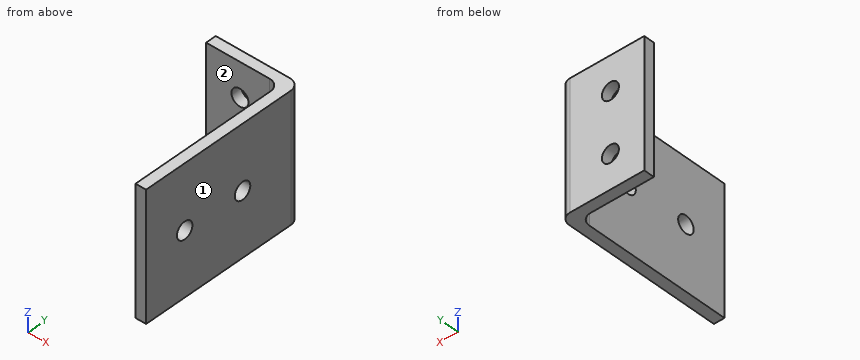
from build123d import *

# Parameters (mm, degrees)
F0_W     = 22.225
F0_H     = 38.1
F0_W_2   = 3.175
F1_DEPTH = 3.175
F2_D     = 5.1054
F3_DEPTH = 50.8
F4_R     = 3.175
F6_D     = 5.1054


with BuildPart() as f1:
    # F0 (on Front) → F1 (new body)
    with BuildSketch(Plane.XZ):
        with Locations((-0.7963004947, 15.9530722331)):
            Rectangle(F0_W, F0_H)
        with Locations((11.9036995053, 15.9530722331)):
            Rectangle(F0_W_2, F0_H)
    extrude(amount=F1_DEPTH)

    # F2 (through all)
    with Locations(Plane(origin=(0, 0, 0), x_dir=(1, 0, 0), z_dir=(0, 1, 0))):
        with Locations((-1.7488004947, -24.8430722331), (-1.7488004947, -7.0630722331)):
            Hole(F2_D / 2)

    # F0 (on Front) → F3 (join)
    with BuildSketch(Plane.XZ):
        with Locations((11.9036995053, 15.9530722331)):
            Rectangle(F0_W_2, F0_H)
    extrude(amount=F3_DEPTH)

    # F4
    f4_edges = [f1.edges().sort_by_distance(p)[0] for p in [
        (10.3162, -3.175, 15.953072),
        (13.4912, 0, 15.953072),
    ]]
    fillet(f4_edges, radius=F4_R)

    # F6 (through all)
    with Locations(Plane(origin=(10.3161995053, 0, 0), x_dir=(0, -1, 0), z_dir=(-1, 0, 0))):
        with Locations((19.05, 15.9530722331), (38.1, 15.9530722331)):
            Hole(F6_D / 2)


solid = f1.part
Model file for the job. Use its own axes, mm. Face numbers are marked on the shaded views. A direction names the side the tool comes from. Round coordinates to 2 decimals unless told otherwise and drop trailing zeros. Order: outer loops, then holes, each group sorted by start corner. A loop starts at its lowest first (then second) coordinate and runs counter-clockwise, first axis right, second up.
(1) Band-saw the part on A-A (y = -38.1). List the corners of the cut face in (x, z), then the cut area to 3 significant figures.
(2) 3-axis set-ups, long thin cutter, end or side, ignore diameter. For the marked faces 1 and 2: which of +Z, -Z, +X, -X, +Y, -Y reach the whole face in a straight line?
(3) Band-saw the part on B-B (x = -0.25). List the corners of the cut face in (y, z) (3 decimals), then the cut area to 3 significant figures.
(4) Band-saw the part on C-C (z = 5.5). List the corners of the cut face in (x, y) (3 decimals), then the cut area to 3 significant figures.
(5) Drill centre lines: line 1 (Z direction, x = 12.1, y = -19.05); line 2 (Y direction, x = 2, z = 8) (3 decimals); line 3 (X direction, y = -32, z = 30.5). Where is each one in solid material? Low to high.
(6) Band-saw the part on D-D (x = 2.75). List the corners of the cut face in (y, z) (3 decimals), then the cut area to 3 significant figures.
(7) Pin check, flat tips, straight feed: pin 1 (11.5 mm diameter, centred on y = -33, z = 12.5, fed in from -X); pin 2 (8 mm diameter, centred on x = 2.5, z = 19, fed in from -Y) (3 decimals); pin 3 (4.5 mm diameter, centred on y = -19.05, z = 15.95, fed in from -X); pin 4 (4 mm diameter, centred on x = 6.5, z = 21.5, fed in from -Y). Stop position of each tip, or through.
Verdict:
1. outline: (10.32, -3.1) - (13.49, -3.1) - (13.49, 13.4) - (10.32, 13.4) - close; (10.32, 18.51) - (13.49, 18.51) - (13.49, 35) - (10.32, 35) - close
1. area: 105 mm2
2. face 1: +Z, -Z, +X, +Y, -Y
2. face 2: +Z, -Z, -X, -Y
3. outline: (-3.175, -3.097) - (0, -3.097) - (0, 4.997) - (-3.175, 4.997) - close; (-3.175, 9.129) - (0, 9.129) - (0, 22.777) - (-3.175, 22.777) - close; (-3.175, 26.909) - (0, 26.909) - (0, 35.003) - (-3.175, 35.003) - close
3. area: 94.7 mm2
4. outline: (-11.909, -3.175) - (-3.767, -3.175) - (-3.767, 0) - (-11.909, 0) - close; (0.269, -3.175) - (7.141, -3.175) arc R3.175 cw to (10.316, -6.35) - (10.316, -50.8) - (13.491, -50.8) - (13.491, -3.175) arc R3.175 ccw to (10.316, 0) - (0.269, 0) - close
4. area: 219 mm2
5. line 1: z = -3.1 to 13.4, 18.51 to 35
5. line 2: y = -3.175 to 0
5. line 3: x = 10.32 to 13.49
6. outline: (-3.175, -3.097) - (0, -3.097) - (0, 35.003) - (-3.175, 35.003) - close
6. area: 121 mm2
7. pin 1: stops at x = 10.32
7. pin 2: stops at y = -3.175
7. pin 3: passes through
7. pin 4: stops at y = -3.48
